```python
from build123d import *

# Parameters (mm, degrees)
SKETCH1_R           = 72.5
BOSS_EXTRUDE1_DEPTH = 384
SKETCH2_R           = 90
BOSS_EXTRUDE2_DEPTH = 10
FILLET1_R           = 10
SKETCH3_R           = 10
BOSS_EXTRUDE3_DEPTH = 40


with BuildPart() as part:
    # Sketch1 → Boss-Extrude1 (new body)
    with BuildSketch(Plane(origin=(0, 0, 0), x_dir=(1, 0, 0), z_dir=(0, 1, 0))):
        Circle(SKETCH1_R)
    extrude(amount=BOSS_EXTRUDE1_DEPTH)

    # Sketch2 → Boss-Extrude2 (add)
    with BuildSketch(Plane(origin=(0, 0, 0), x_dir=(1, 0, 0), z_dir=(0, 1, 0))):
        Circle(SKETCH2_R)
    extrude(amount=BOSS_EXTRUDE2_DEPTH)

    # Fillet1
    fillet1_edges = [part.edges().sort_by_distance(p)[0] for p in [
        (-72.5, 10, 0),
    ]]
    fillet(fillet1_edges, radius=FILLET1_R)

    # Sketch3 → Boss-Extrude3 (add)
    with BuildSketch(Plane(origin=(0, 384, 0), x_dir=(1, 0, 0), z_dir=(0, 1, 0))):
        Circle(SKETCH3_R)
    extrude(amount=BOSS_EXTRUDE3_DEPTH)


solid = part.part
```
The listing builds one solid part. Answer for the finished solid, in the listing's coordinates (mm). A direction names the side the tool comes from. Give positions to 0.01 mm unless a question says otherwise; leave off trailing zeros. Write each loop counter-clockwise with the first axis right and the second up, starting at its lowest first coordinate (ties: lowest second). Pieces come first, ordered by that corner, then holes. Notation, with made-up numbers: (-32, 5.25) - (-15, 5.25) arc R24 ccw to (-15, 39.25) - close; hole circle Ø7 at (88, -33). An arc over 180 degrees is marked (long way). Use one line per item in the form item = value. Start each with the question number.
1) Consider line 1 along Y through (x, z) = (0.5, -35.5); line 2 along Y through (x, z) = (34, 82); line 3 along Z through (x, y) = (-0.5, 365). Determine where each line is inside the solid, lowest interval first. Write a range as from..to.
2) Find section C-C on y = 181. Determine the outline of the cut face in (x, z), plus the area to 3 significant figures.
3) A tool of negligible diameter and unlimited length cuts with its end or side. For faces 1 (the face through (-2.17, 403.72, 9.76)), 2 (the face through (0, 424, 0)), from which of +Z, -Z, +X, -X, +Y, -Y can it reach the whole face along a straight path? Write none if from no direction.
4) Find section B-B on x = 0. Determine the outline of the cut face in (y, z).
5) Flat-ended cylindrical pins translate along their axes: pin 1 Ø5 at (x, y) = (-38.5, 210.5) entering from +Z; pin 2 Ø6 at (y, z) = (347, -49) entering from -X; pin 3 Ø10 at (y, z) = (190, 55.5) entering from -X; pin 4 Ø8 at (x, z) = (-24, -38) entering from -Y. Find the tip coordinate at first contact, or state that the pin passes through.
6) Find section A-A on z = 0. Determine the outline of the cut face in (x, y), plus the area to 3 significant figures.
Geometry results:
q1.line_1 = 0..384
q1.line_2 = 0..10
q1.line_3 = -72.5..72.5
q2.outline = circle Ø145 at (0, 0)
q2.area = 16,500 mm2
q3.face_1 = +Y
q3.face_2 = +Z, -Z, +X, -X, +Y
q4.outline = (0, -90) - (10, -90) - (10, -82.5) arc R10 cw to (20, -72.5) - (384, -72.5) - (384, -10) - (424, -10) - (424, 10) - (384, 10) - (384, 72.5) - (20, 72.5) arc R10 cw to (10, 82.5) - (10, 90) - (0, 90) - close
q5.pin_1 = 62.93
q5.pin_2 = -56.04
q5.pin_3 = -52.02
q5.pin_4 = 0
q6.outline = (-90, 0) - (90, 0) - (90, 10) - (82.5, 10) arc R10 cw to (72.5, 20) - (72.5, 384) - (10, 384) - (10, 424) - (-10, 424) - (-10, 384) - (-72.5, 384) - (-72.5, 20) arc R10 cw to (-82.5, 10) - (-90, 10) - close
q6.area = 56,900 mm2
